```python
from build123d import *

# Parameters (mm, degrees)
SKETCH1_R           = 7.8105
BOSS_EXTRUDE1_DEPTH = 15.113
SKETCH2_W           = 14.883103562
SKETCH2_H           = 1.269889382
CUT_EXTRUDE1_DEPTH  = 19.719257183
BOSS_EXTRUDE2_START = -5.08
SKETCH3_R           = 9.2075
BOSS_EXTRUDE2_DEPTH = 2.1336


with BuildPart() as part:
    # Sketch1 → Boss-Extrude1 (new body)
    with BuildSketch(Plane.XY):
        Circle(SKETCH1_R)
    extrude(amount=BOSS_EXTRUDE1_DEPTH)

    # Sketch2 → Cut-Extrude1 (cut, through all)
    with BuildSketch(Plane.XY.offset(15.113)):
        with Locations((0, 7.975544691)):
            Rectangle(SKETCH2_W, SKETCH2_H)
        with Locations((0, -7.975544691)):
            Rectangle(SKETCH2_W, SKETCH2_H)
    extrude(amount=-CUT_EXTRUDE1_DEPTH, mode=Mode.SUBTRACT)

    # Sketch3 → Boss-Extrude2 (add)
    with BuildSketch(Plane(origin=(0, 0, 0), x_dir=(-1, 0, 0), z_dir=(0, 0, -1)).offset(BOSS_EXTRUDE2_START)):
        Circle(SKETCH3_R)
    extrude(amount=-BOSS_EXTRUDE2_DEPTH)


solid = part.part
```
Geometry check sheet. Reference: the model listing, model coordinates, mm. A direction names the side the tool comes from. Give positions to 0.01 mm unless a question says otherwise; leave off trailing zeros. Loops run counter-clockwise (first coordinate to the right, second up) from the corner with the lowest first, then second, coordinate; pieces in that order, holes last. Notation, with made-up numbers: M 87,27 L 95,27 A15 cw 95,38 Z; hole C 63,53.25 d8. An arc over 180 degrees is marked long. Answer as CSV lines item,"result".
Item 1: Cross-section at D-D on z = 13.5. Record the cut outline in (x, y).
Values:
outline,"M -2.67,-7.34 L 2.67,-7.34 A7.81 ccw 2.67,7.34 L -2.67,7.34 A7.81 ccw Z"
Item 2: Cross-section at B-B on y = 0. Record the cut outline in (x, z), and give its area (3 significant figures).
Values:
outline,"M -9.21,5.08 L -7.81,5.08 L -7.81,0 L 7.81,0 L 7.81,5.08 L 9.21,5.08 L 9.21,7.21 L 7.81,7.21 L 7.81,15.11 L -7.81,15.11 L -7.81,7.21 L -9.21,7.21 Z"
area,"242 mm²"
Item 3: Material ranges on line 1 (Y direction, x = -1.75, z = 13); line 2 (Z direction, x = -4.75, y = 7); line 3 (X direction, y = 0.75, z = 11), recorded low to high.
Values:
line 1,"y = -7.34 to 7.34"
line 2,"z = 5.08 to 7.21"
line 3,"x = -7.77 to 7.77"
Item 4: Cross-section at A-A on x = 0. Record the cut outline in (y, z).
Values:
outline,"M -9.21,5.08 L -7.34,5.08 L -7.34,0 L 7.34,0 L 7.34,5.08 L 9.21,5.08 L 9.21,7.21 L 7.34,7.21 L 7.34,15.11 L -7.34,15.11 L -7.34,7.21 L -9.21,7.21 Z"
Item 5: Access from +Z, -Z, +X, -X, +Y, -Y to the whole of each face (thin tool, end or side, straight path). Record for faces 1 (the cylindrical face through (-7.81, 0.13, 2.5)), 2 (the cylindrical face through (-7.81, 0.13, 11.11)), 3 (the flat face through (0, -7.5, 5.08)), 4 (the flat face through (0, -7.5, 7.214)).
Values:
face 1,"-Z, -X"
face 2,"+Z, -X"
face 3,"-Z"
face 4,"+Z"
Item 6: Cross-section at C-C on z = 6.5. Record the cut outline in (x, y) (1 decimal), and give its area (3 significant figures).
Values:
outline,"C 0,0 d18.4"
area,"266 mm²"
Item 7: Depth check by flat-ended pin: P1, Ø1, axis at y = -6.5, z = 7, coming from the -X side; P2, Ø4.5, axis at x = -1, z = 12.5, coming from the -Y side; P3, Ø2, axis at y = 3.5, z = 10, coming from the +X side. Enter the tip coordinate at first touch or a pass-through.
Values:
P1,"stops at x = -6.98"
P2,"stops at y = -7.34"
P3,"stops at x = 7.4"
